```python
from build123d import *

# Parameters (mm, degrees)
F0_W     = 21.2
F0_H     = 18
F1_DEPTH = 8.4
F2_W     = 19.2
F2_H     = 16
F3_DEPTH = 7.5
F4_W     = 25.2
F4_H     = 24
F4_W_2   = 21.2
F4_H_2   = 18
F5_DEPTH = 1
F6_R     = 1.2
F7_DEPTH = 0.901


with BuildPart() as f1:
    # F0 (on Top) → F1 (new body)
    with BuildSketch(Plane.XY):
        with Locations((10.6, 9)):
            Rectangle(F0_W, F0_H)
    extrude(amount=F1_DEPTH)

    # F2 (on face) → F3 (cut)
    with BuildSketch(Plane.XY.offset(8.4)):
        with Locations((10.6, 9)):
            Rectangle(F2_W, F2_H)
    extrude(amount=-F3_DEPTH, mode=Mode.SUBTRACT)

    # F4 (on face) → F5 (join)
    with BuildSketch(Plane.XY.offset(8.4)):
        with Locations((10.6, 10)):
            Rectangle(F4_W, F4_H)
        with Locations((10.6, 9)):
            Rectangle(F4_W_2, F4_H_2, mode=Mode.SUBTRACT)
    extrude(amount=-F5_DEPTH)

    # F6 (on face) → F7 (cut, through all)
    with BuildSketch(Plane.XY.offset(0.9)):
        with Locations((10.6, 8)):
            Circle(F6_R)
    extrude(amount=-F7_DEPTH, mode=Mode.SUBTRACT)


solid = f1.part
```
Here's how the part is built. I have some questions about the finished solid (model axes, mm). A direction names the side the tool comes from. Coordinates: 2 decimals unless noted, no trailing zeros. Order: outer loops, then holes, each group sorted by start corner. A loop starts at its lowest first (then second) coordinate and runs counter-clockwise, first axis right, second up.
1) I need wall thicknesses on line 1 (Y direction, x = 6, z = 3); line 2 (X direction, y = 11.75, z = 5.75); line 3 (X direction, y = 2.5, z = 8). Which ranges of each line are inside material? Lowest first, please.
2) Imagine slicing it at B-B on y = 8. List the corners of the cut face in (x, z) for me.
3) Imagine slicing it at D-D on y = 17.5. List the corners of the cut face in (x, z) for me, and give its area (3 significant figures).
4) Imagine slicing it at C-C on z = 2.5. List the corners of the cut face in (x, y) for me, and give its area (3 significant figures).
5) We'd pull the mould along Y, two halves only. Please class faces 1 (the face through (10, 0, 4)), 2 (the face through (10, 11, 0.9)), 3 (the face through (-2, 10, 8)): +Y half, -Y half, draft (parallel to the pull), parting line (faces both ways), or undercut.
6) Will these pins go through, and if not, where does the flat tip stop? pin 1 (3 mm diameter, centred on y = 5, z = 3, fed in from -X); pin 2 (2 mm diameter, centred on x = 12, z = 3, fed in from -Y); pin 3 (1 mm diameter, centred on y = 10.5, z = 3, fed in from +X); pin 4 (3 mm diameter, centred on x = 12, z = 6.5, fed in from -Y).
7) Imagine slicing it at A-A on x = 10.6. List the corners of the cut face in (y, z) for me, and give its area (3 significant figures).
8) Which directions (+Z, -Z, +X, -X, +Y, -Y) give clear straight access to the entire face, cutting with the end or side of a thin tool? Please do faces 4 (the face through (21.2, 9, 4)), 5 (the face through (10, 18, 4)), 6 (the face through (10, -2, 8)), 7 (the face through (10, 1, 5)), 8 (the face through (0, 9, 4)).
Response values:
1. line 1: y = 0 to 1, 17 to 18
1. line 2: x = 0 to 1, 20.2 to 21.2
1. line 3: x = -2 to 1, 20.2 to 23.2
2. outline: (-2, 7.4) - (0, 7.4) - (0, 0) - (9.4, 0) - (9.4, 0.9) - (1, 0.9) - (1, 8.4) - (-2, 8.4) - close; (11.8, 0) - (21.2, 0) - (21.2, 7.4) - (23.2, 7.4) - (23.2, 8.4) - (20.2, 8.4) - (20.2, 0.9) - (11.8, 0.9) - close
3. outline: (-2, 7.4) - (0, 7.4) - (0, 0) - (21.2, 0) - (21.2, 7.4) - (23.2, 7.4) - (23.2, 8.4) - (-2, 8.4) - close
3. area: 182 mm2
4. outline: (0, 0) - (21.2, 0) - (21.2, 18) - (0, 18) - close; hole (1, 1) - (20.2, 1) - (20.2, 17) - (1, 17) - close
4. area: 74.4 mm2
5. face 1: -Y half
5. face 2: undercut
5. face 3: draft
6. pin 1: stops at x = 0
6. pin 2: stops at y = 0
6. pin 3: stops at x = 21.2
6. pin 4: stops at y = -2
7. outline: (-2, 7.4) - (0, 7.4) - (0, 0) - (6.8, 0) - (6.8, 0.9) - (1, 0.9) - (1, 8.4) - (-2, 8.4) - close; (9.2, 0) - (18, 0) - (18, 7.4) - (22, 7.4) - (22, 8.4) - (17, 8.4) - (17, 0.9) - (9.2, 0.9) - close
7. area: 35.0 mm2
8. face 4: -Z, +X, +Y, -Y
8. face 5: -Z, +X, -X, +Y
8. face 6: +Z, -Z, +X, -X, -Y
8. face 7: +Z
8. face 8: -Z, -X, +Y, -Y
